Design review of the part built by this model. Coordinates are the model's own, in mm. Give positions to 0.01 mm unless a question says otherwise; leave off trailing zeros. Loops run counter-clockwise (first coordinate to the right, second up) from the corner with the lowest first, then second, coordinate; pieces in that order, holes last.
from build123d import *

# Parameters (mm, degrees)
SKETCH2_R           = 51.054
SKETCH2_R_2         = 49.53
BOSS_EXTRUDE1_DEPTH = 508
SKETCH3_R           = 1.524
CUT_EXTRUDE1_DEPTH  = 74.422
CIRPATTERN1_COUNT   = 6
SKETCH4_R           = 1.524
CUT_EXTRUDE2_DEPTH  = 74.422
CIRPATTERN2_COUNT   = 6


with BuildPart() as part:
    # Sketch2 → Boss-Extrude1 (new body)
    with BuildSketch(Plane(origin=(0, 0, 0), x_dir=(1, 0, 0), z_dir=(0, 1, 0))):
        with Locations(Location((0, 0, 0), (0, 0, 270))):
            Circle(SKETCH2_R)
        with Locations(Location((0, 0, 0), (0, 0, 270))):
            Circle(SKETCH2_R_2, mode=Mode.SUBTRACT)
    extrude(amount=BOSS_EXTRUDE1_DEPTH)

    # Sketch3 → Cut-Extrude1 (cut)
    with BuildSketch(Plane.XY):
        with Locations(Location((0, 393.7, 0), (0, 0, 90))):
            Circle(SKETCH3_R)
    cut_extrude1 = extrude(amount=-CUT_EXTRUDE1_DEPTH, mode=Mode.SUBTRACT)

    # CirPattern1: Cut-Extrude1 ×6 about axis
    cirpattern1_axis = Axis((0, 508, 0), (0, -1, 0))
    for i in range(1, CIRPATTERN1_COUNT):
        add(cut_extrude1.rotate(cirpattern1_axis, i * 360 / CIRPATTERN1_COUNT), mode=Mode.SUBTRACT)

    # Sketch4 → Cut-Extrude2 (cut)
    with BuildSketch(Plane(origin=(0, 0, 0), x_dir=(0, 0, -1), z_dir=(1, 0, 0))):
        with Locations((0, 19.05)):
            Circle(SKETCH4_R)
    cut_extrude2 = extrude(amount=-CUT_EXTRUDE2_DEPTH, mode=Mode.SUBTRACT)

    # CirPattern2: Cut-Extrude2 ×6 about axis
    cirpattern2_axis = Axis((0, 508, 0), (0, -1, 0))
    for i in range(1, CIRPATTERN2_COUNT):
        add(cut_extrude2.rotate(cirpattern2_axis, i * 360 / CIRPATTERN2_COUNT), mode=Mode.SUBTRACT)


solid = part.part
Q1. Insertion check: pin 1 (4 mm diameter, centred on x = -25.5, y = 254, fed in from -Z); pin 2 (2.5 mm diameter, centred on y = 19.05, z = 0, fed in from +X); pin 3 (6 mm diameter, centred on x = 9.5, y = 175, fed in from +Z); pin 4 (2 mm diameter, centred on y = 207, z = 4.5, fed in from -X). Each pin has a flat end and moves straight along its axis. Give the tip position at first contact, or say it passes through.
Results:
pin 1: stops at z = -45.32
pin 2: passes through
pin 3: stops at z = 50.64
pin 4: stops at x = -50.93
Q2. Take a section at A-A (y = 402.5). Give the boundary of the cut face in (x, z).
Results:
outline: circle Ø102.11 at (0, 0); hole circle Ø99.06 at (0, 0)
Q3. Wall thickness on line 1 (Y direction, x = 49.9, z = 0); line 2 (X direction, y = 296, z = 0); line 3 (Z direction, x = 2, y = 321): over which ranges is each line inside the solid? List them lowest first.
Results:
line 1: y = 0 to 17.53, 20.57 to 508
line 2: x = -51.05 to -49.53, 49.53 to 51.05
line 3: z = -51.01 to -49.49, 49.49 to 51.01
Q4. Draft analysis for pull direction X (two halves, no side actions). For faces 1 (the face through (-19.554, 250.444, 47.161)), 2 (the face through (27, 508, -42)), 3 (the face through (14.88, 250.44, 47.24)), state which applies: pulls with the +X half, pulls with the -X half, needs draft (parallel to the pull), parting line crosses it, or undercut.
Results:
face 1: parting line crosses it
face 2: needs draft
face 3: undercut
